from build123d import *

# Parameters (mm, degrees)
ESQUISSE1_W             = 80
ESQUISSE1_H             = 20
BOSS_EXTRU_1_DEPTH      = 15
ENL_V_MAT_EXTRU_1_DEPTH = 94
ESQUISSE3_R             = 2.5
ENL_V_MAT_EXTRU_2_DEPTH = 94


with BuildPart() as part:
    # Esquisse1 → Boss.-Extru.1 (new body)
    with BuildSketch(Plane.XY):
        with Locations((-40, 10)):
            Rectangle(ESQUISSE1_W, ESQUISSE1_H)
    extrude(amount=BOSS_EXTRU_1_DEPTH)

    # Esquisse2 → Enlèv. mat.-Extru.1 (cut)
    with BuildSketch(Plane(origin=(0, 0, 0), x_dir=(0, 0, -1), z_dir=(1, 0, 0))):
        with BuildLine():
            Line((-15, 7.5), (-10, 7.5))
            ThreePointArc((-10, 7.5), (-7.5, 10), (-10, 12.5))
            Line((-10, 12.5), (-15, 12.5))
            Line((-15, 12.5), (-15, 7.5))
        make_face()
    extrude(amount=-ENL_V_MAT_EXTRU_1_DEPTH, mode=Mode.SUBTRACT)

    # Esquisse3 → Enlèv. mat.-Extru.2 (cut)
    with BuildSketch(Plane(origin=(0, 0, 0), x_dir=(-1, 0, 0), z_dir=(0, 0, -1))):
        with Locations((10, 17)):
            Circle(ESQUISSE3_R)
        with Locations((10, 3)):
            Circle(ESQUISSE3_R)
        with Locations((70, 17)):
            Circle(ESQUISSE3_R)
        with Locations((70, 3)):
            Circle(ESQUISSE3_R)
    extrude(amount=-ENL_V_MAT_EXTRU_2_DEPTH, mode=Mode.SUBTRACT)


solid = part.part
Build history of the part. All positions in model axes, mm. A direction names the side the tool comes from. Give positions to 0.01 mm unless a question says otherwise; leave off trailing zeros. Order: outer loops, then holes, each group sorted by start corner. A loop starts at its lowest first (then second) coordinate and runs counter-clockwise, first axis right, second up. Notation, with made-up numbers: M 84.25,31 L 126.25,31 A33 ccw 126.25,62 Z; hole C 76.25,56.5 d1. An arc over 180 degrees is marked long. Use one line per item in the form item = value.
Q1. Pull direction X, two halves, no side cores. Call faces 1 (the flat face through (0, 10, 7)), 2 (the cylindrical face through (-9.46, 0.56, 7.4)), 3 (the flat face through (-41, 4, 15)): released by +X, released by -X, zero draft, split by the parting line, or undercut.
Conclusion:
face_1 = released by +X
face_2 = undercut
face_3 = zero draft
Q2. Slice it at B-B, the plane y = 17. Write the cut outline in (x, z), and give its area (3 significant figures).
Conclusion:
outline = M -80,0 L -72.5,0 L -72.5,15 L -80,15 Z; M -67.5,0 L -12.5,0 L -12.5,15 L -67.5,15 Z; M -7.5,0 L 0,0 L 0,15 L -7.5,15 Z
area = 1,050 mm2
Q3. Which spindle directions (+Z, -Z, +X, -X, +Y, -Y) get a long thin tool onto all of the face, cutting with end or side? Do faces 4 (the flat face through (-41, 0, 7)), 5 (the flat face through (-39, 7.5, 13)). Say none if no direction does.
Conclusion:
face_4 = +Z, -Z, +X, -X, -Y
face_5 = +Z, +X, -X
Q4. Slice it at D-D, the plane z = 1. Write the cut outline in (x, y).
Conclusion:
outline = M -80,0 L 0,0 L 0,20 L -80,20 Z; hole C -70,3 d5; hole C -70,17 d5; hole C -10,3 d5; hole C -10,17 d5
Q5. Wall check: probe 1 along Y at (x, z) = (-10, 11.75); probe 2 along Y at (x, z) = (-70, 4.5); probe 3 along X at (y, z) = (18, 3). Give the ranges that are in metal, low to high.
Conclusion:
probe_1 = 0 to 0.5, 5.5 to 7.5, 12.5 to 14.5, 19.5 to 20
probe_2 = 0 to 0.5, 5.5 to 14.5, 19.5 to 20
probe_3 = -80 to -72.29, -67.71 to -12.29, -7.71 to 0
Q6. Slice it at C-C, the plane z = 11.75. Write the cut outline in (x, y).
Conclusion:
outline = M -80,0 L 0,0 L 0,7.5 L -80,7.5 Z; M -80,12.5 L 0,12.5 L 0,20 L -80,20 Z; hole C -70,3 d5; hole C -70,17 d5; hole C -10,3 d5; hole C -10,17 d5
Q7. Slice it at A-A, the plane x = -70. Write the cut outline in (y, z), and give its area (3 significant figures).
Conclusion:
outline = M 0,0 L 0.5,0 L 0.5,15 L 0,15 Z; M 5.5,0 L 14.5,0 L 14.5,15 L 12.5,15 L 12.5,10 A2.5 cw 7.5,10 L 7.5,15 L 5.5,15 Z; M 19.5,0 L 20,0 L 20,15 L 19.5,15 Z
area = 115 mm2
